```python
from build123d import *
from build123d import SkipClean  # not in build123d's __all__

# Parameters (mm, degrees)
F0_R     = 0.8
F1_DEPTH = 6.4
F2_DEPTH = 1
F3_DEPTH = 4.1
F4_W     = 0.5
F4_H     = 15
F5_DEPTH = 25
F7_D     = 3.3
F7_DEPTH = 3.2
F7_TIP   = 0.9914200214
F8_D     = 2.4
F8_DEPTH = 3.5
F8_TIP   = 0.7210327428


with BuildPart() as f1:
    # F0 (on Top) → F1 (new body)
    with BuildSketch(Plane.XY):
        with BuildLine():
            Line((-24, -3.2), (-1.4177446879, -3.2))
            ThreePointArc((-1.4177446879, -3.2), (-2.4227036384, -2.5259665636), (-3.1380726569, -1.55))
            ThreePointArc((-3.1380726569, -1.55), (-3.5, 0), (-3.1380726569, 1.55))
            ThreePointArc((-3.1380726569, 1.55), (-2.4227036384, 2.5259665636), (-1.4177446879, 3.2))
            Line((-1.4177446879, 3.2), (-24, 3.2))
            Line((-24, 3.2), (-24, -3.2))
        make_face()
        with Locations((-21.5, 0)):
            Circle(F0_R, mode=Mode.SUBTRACT)
        with Locations((-18, 0)):
            Circle(F0_R, mode=Mode.SUBTRACT)
        with Locations((-14.5, 0)):
            Circle(F0_R, mode=Mode.SUBTRACT)
        with Locations((-11, 0)):
            Circle(F0_R, mode=Mode.SUBTRACT)
        with Locations((-7.5, 0)):
            Circle(F0_R, mode=Mode.SUBTRACT)
        with BuildLine():
            Line((-3.1380726569, -1.55), (-1.3416407865, -1.55))
            ThreePointArc((-1.3416407865, -1.55), (-2.05, 0), (-1.3416407865, 1.55))
            Line((-1.3416407865, 1.55), (-3.1380726569, 1.55))
            ThreePointArc((-3.1380726569, 1.55), (-3.5, 0), (-3.1380726569, -1.55))
        make_face()
        with BuildLine():
            ThreePointArc((1.4177446879, -3.2), (2.4227036384, -2.5259665636), (3.1380726569, -1.55))
            Line((3.1380726569, -1.55), (1.3416407865, -1.55))
            ThreePointArc((1.3416407865, -1.55), (0, -2.05), (-1.3416407865, -1.55))
            Line((-1.3416407865, -1.55), (-3.1380726569, -1.55))
            ThreePointArc((-3.1380726569, -1.55), (-2.4227036384, -2.5259665636), (-1.4177446879, -3.2))
            Line((-1.4177446879, -3.2), (1.4177446879, -3.2))
        make_face()
        with BuildLine():
            Line((1.3416407865, 1.55), (3.1380726569, 1.55))
            ThreePointArc((3.1380726569, 1.55), (2.4227036384, 2.5259665636), (1.4177446879, 3.2))
            Line((1.4177446879, 3.2), (-1.4177446879, 3.2))
            ThreePointArc((-1.4177446879, 3.2), (-2.4227036384, 2.5259665636), (-3.1380726569, 1.55))
            Line((-3.1380726569, 1.55), (-1.3416407865, 1.55))
            ThreePointArc((-1.3416407865, 1.55), (0, 2.05), (1.3416407865, 1.55))
        make_face()
        with BuildLine():
            ThreePointArc((1.3416407865, 1.55), (0, 2.05), (-1.3416407865, 1.55))
            Line((-1.3416407865, 1.55), (1.3416407865, 1.55))
        make_face()
        with BuildLine():
            ThreePointArc((-1.3416407865, -1.55), (0, -2.05), (1.3416407865, -1.55))
            Line((1.3416407865, -1.55), (-1.3416407865, -1.55))
        make_face()
        with BuildLine():
            Line((1.3416407865, -1.55), (3.1380726569, -1.55))
            ThreePointArc((3.1380726569, -1.55), (3.4083173487, -0.7958472532), (3.5, 0))
            ThreePointArc((3.5, 0), (3.4083173487, 0.7958472532), (3.1380726569, 1.55))
            Line((3.1380726569, 1.55), (1.3416407865, 1.55))
            ThreePointArc((1.3416407865, 1.55), (1.864519189, 0.8520963524), (2.05, 0))
            ThreePointArc((2.05, 0), (1.864519189, -0.8520963524), (1.3416407865, -1.55))
        make_face()
        with BuildLine():
            ThreePointArc((3.5, 0), (3.4083173487, -0.7958472532), (3.1380726569, -1.55))
            ThreePointArc((3.1380726569, -1.55), (2.4227036384, -2.5259665636), (1.4177446879, -3.2))
            Line((1.4177446879, -3.2), (10, -3.2))
            Line((10, -3.2), (10, 3.2))
            Line((10, 3.2), (1.4177446879, 3.2))
            ThreePointArc((1.4177446879, 3.2), (2.4227036384, 2.5259665636), (3.1380726569, 1.55))
            ThreePointArc((3.1380726569, 1.55), (3.4083173487, 0.7958472532), (3.5, 0))
        make_face()
        with BuildLine():
            ThreePointArc((-1.4177446879, -3.2), (0, -3.5), (1.4177446879, -3.2))
            Line((1.4177446879, -3.2), (-1.4177446879, -3.2))
        make_face()
        with BuildLine():
            Line((-1.4177446879, 3.2), (1.4177446879, 3.2))
            ThreePointArc((1.4177446879, 3.2), (0, 3.5), (-1.4177446879, 3.2))
        make_face()
    extrude(amount=F1_DEPTH)

    # F0 (on Top) → F2 (cut)
    with BuildSketch(Plane.XY):
        with BuildLine():
            ThreePointArc((3.5, 0), (3.4083173487, -0.7958472532), (3.1380726569, -1.55))
            ThreePointArc((3.1380726569, -1.55), (2.4227036384, -2.5259665636), (1.4177446879, -3.2))
            Line((1.4177446879, -3.2), (10, -3.2))
            Line((10, -3.2), (10, 3.2))
            Line((10, 3.2), (1.4177446879, 3.2))
            ThreePointArc((1.4177446879, 3.2), (2.4227036384, 2.5259665636), (3.1380726569, 1.55))
            ThreePointArc((3.1380726569, 1.55), (3.4083173487, 0.7958472532), (3.5, 0))
        make_face()
    with SkipClean():  # cleaning this boolean's faces spoils the solid; the shape is the same uncleaned
        extrude(amount=F2_DEPTH, mode=Mode.SUBTRACT)

    # F0 (on Top) → F3 (cut)
    with BuildSketch(Plane.XY):
        with BuildLine():
            Line((-24, -3.2), (-1.4177446879, -3.2))
            ThreePointArc((-1.4177446879, -3.2), (-2.4227036384, -2.5259665636), (-3.1380726569, -1.55))
            ThreePointArc((-3.1380726569, -1.55), (-3.5, 0), (-3.1380726569, 1.55))
            ThreePointArc((-3.1380726569, 1.55), (-2.4227036384, 2.5259665636), (-1.4177446879, 3.2))
            Line((-1.4177446879, 3.2), (-24, 3.2))
            Line((-24, 3.2), (-24, -3.2))
        make_face()
        with Locations((-21.5, 0)):
            Circle(F0_R, mode=Mode.SUBTRACT)
        with Locations((-18, 0)):
            Circle(F0_R, mode=Mode.SUBTRACT)
        with Locations((-14.5, 0)):
            Circle(F0_R, mode=Mode.SUBTRACT)
        with Locations((-11, 0)):
            Circle(F0_R, mode=Mode.SUBTRACT)
        with Locations((-7.5, 0)):
            Circle(F0_R, mode=Mode.SUBTRACT)
    extrude(amount=F3_DEPTH, mode=Mode.SUBTRACT)

    # F4 (on Right) → F5 (cut)
    with BuildSketch(Plane.YZ):
        Rectangle(F4_W, F4_H)
    extrude(amount=F5_DEPTH, mode=Mode.SUBTRACT)

    # F7 (one way)
    with BuildSketch(Plane(origin=(0, 0, 0), x_dir=(1, 0, 0), z_dir=(0, 1, 0))):
        with Locations((7, -3.7)):
            Circle(F7_D / 2)
    extrude(amount=-F7_DEPTH, mode=Mode.SUBTRACT)
    with Locations(Plane(origin=(0, 0, 0), x_dir=(1, 0, 0), z_dir=(0, 1, 0))):
        with Locations((7, -3.7)):
            with Locations((0, 0, -(F7_DEPTH + F7_TIP / 2))):  # 118° drill point
                Cone(0, F7_D / 2, F7_TIP, mode=Mode.SUBTRACT)

    # F8
    with Locations(Plane.XZ):
        with Locations((7, 3.7)):
            Hole(F8_D / 2, depth=F8_DEPTH)
            with Locations((0, 0, -(F8_DEPTH + F8_TIP / 2))):  # 118° drill point
                Cone(0, F8_D / 2, F8_TIP, mode=Mode.SUBTRACT)


solid = f1.part
```
Check sheet for the modelled part. Datum: model origin and axes. Units: mm. A direction names the side the tool comes from. Round coordinates to 2 decimals unless told otherwise and drop trailing zeros. Loops run counter-clockwise (first coordinate to the right, second up) from the corner with the lowest first, then second, coordinate; pieces in that order, holes last. Notation, with made-up numbers: (63, 26.5) -> (104, 26.5) arc R31 ccw to (104, 56.5) -> close; hole circle Ø6 at (57, 74.5). An arc over 180 degrees is marked (long way). Answer in a Markdown table with one row per item.
Q1. Thickness scan on L1, parallel to Y at x = -14.5, z = 5.6; L2, parallel to X at y = -1.25, z = 2.5; L3, parallel to Y at x = 5, z = 6. Record the ranges inside material, lowest first.
Data:
| item | result |
|---|---|
| L1 | y = -3.2 to -0.8, 0.8 to 3.2 |
| L2 | x = -3.27 to -1.62, 1.62 to 5.87, 8.13 to 10 |
| L3 | y = -3.2 to -0.25, 0.25 to 3.2 |
Q2. Set-up check for faces 5 (the face through (5.77, 3.2, 3.06)), 6 (the face through (1.81, -0.96, 3.16)), 7 (the face through (-13, -3.2, 5)), 8 (the face through (5, -0.25, 3)), 9 (the face through (-13, 3.2, 5)): record each of +Z, -Z, +X, -X, +Y, -Y from which the full face is reachable in a straight line by a thin tool's end or side.
Data:
| item | result |
|---|---|
| face 5 | +Z, -Z, +X, +Y |
| face 6 | +Z, -Z |
| face 7 | +Z, -Z, -X, -Y |
| face 8 | +Z, -Z, +X |
| face 9 | +Z, -Z, -X, +Y |
Q3. Sectioned sample at A-A on z = 3.7. Enter the section's corners in (x, y), then the cut area to 3 significant figures.
Data:
| item | result |
|---|---|
| outline | (-1.34, -1.55) arc R2.05 cw to (-1.34, 1.55) -> (1.34, 1.55) arc R2.05 cw to (2.03, 0.25) -> (5.8, 0.25) -> (5.8, 3.2) -> (1.42, 3.2) arc R3.5 ccw (long way) to (1.42, -3.2) -> (5.35, -3.2) -> (5.35, -0.25) -> (2.03, -0.25) arc R2.05 cw to (1.34, -1.55) -> close; (8.2, 0.25) -> (10, 0.25) -> (10, 3.2) -> (8.2, 3.2) -> close; (8.65, -3.2) -> (10, -3.2) -> (10, -0.25) -> (8.65, -0.25) -> close |
| area | 51.7 mm^2 |
Q4. Sectioned sample at D-D on y = 2.75. Enter the section's corners in (x, z).
Data:
| item | result |
|---|---|
| outline | (-24, 4.1) -> (-2.17, 4.1) -> (-2.17, 0) -> (2.17, 0) -> (2.17, 1) -> (10, 1) -> (10, 6.4) -> (-24, 6.4) -> close; hole circle Ø2.4 at (7, 3.7) |
Q5. Sectioned sample at C-C on x = -14.5. Enter the section's corners in (y, z).
Data:
| item | result |
|---|---|
| outline | (-3.2, 4.1) -> (-0.8, 4.1) -> (-0.8, 6.4) -> (-3.2, 6.4) -> close; (0.8, 4.1) -> (3.2, 4.1) -> (3.2, 6.4) -> (0.8, 6.4) -> close |
Q6. Sectioned sample at B-B on x = 7. Enter the section's corners in (y, z).
Data:
| item | result |
|---|---|
| outline | (-3.2, 1) -> (-0.25, 1) -> (-0.25, 2.05) -> (-3.2, 2.05) -> close; (-3.2, 5.35) -> (-0.25, 5.35) -> (-0.25, 6.4) -> (-3.2, 6.4) -> close; (0.25, 1) -> (3.2, 1) -> (3.2, 2.5) -> (0.25, 2.5) -> close; (0.25, 4.9) -> (3.2, 4.9) -> (3.2, 6.4) -> (0.25, 6.4) -> close |
Q7. Go/stop test with flat-tipped pins: P1, Ø2.5, axis at x = -11.5, z = 5, coming from the -Y side; P2, Ø3, axis at x = 7.5, y = 2, coming from the -Z side; P3, Ø1.6, axis at x = 5.5, z = 5, coming from the +Y side; P4, Ø1, axis at x = -18, y = 0, coming from the -Z side. Record where each tip stops, or that it passes through.
Data:
| item | result |
|---|---|
| P1 | stops at y = -3.2 |
| P2 | stops at z = 1 |
| P3 | stops at y = 3.2 |
| P4 | passes through |
Q8. Release check for a two-part mould opening along X. For faces 1 (the face through (-8.3, 0, 5.2)), 2 (the face through (5, -3.2, 4)), 3 (the face through (10, -2, 4)), 4 (the face through (5.69, -1.7, 4.7)) record: released by +X, released by -X, zero draft, split by the parting line, or undercut.
Data:
| item | result |
|---|---|
| face 1 | undercut |
| face 2 | zero draft |
| face 3 | released by +X |
| face 4 | undercut |
